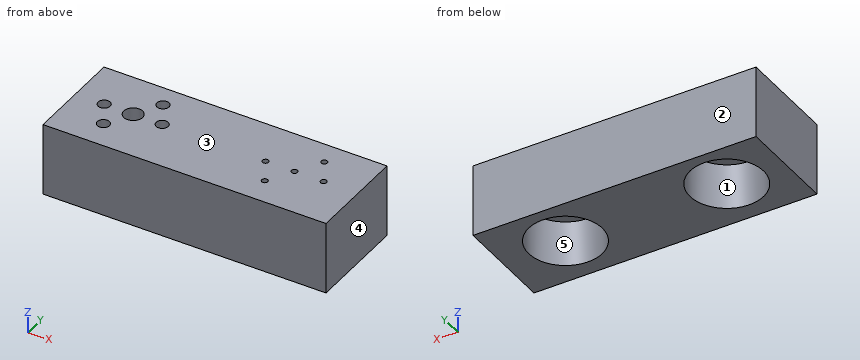
Autodesk Inventor part; units mm, degrees
ref_plane "YZ Plane" through (0, 0, 0) normal (1, 0, 0) x (0, 1, 0)
ref_plane "XZ Plane" through (0, 0, 0) normal (0, 1, 0) x (-1, 0, 0)
ref_plane "XY Plane" through (0, 0, 0) normal (0, 0, 1) x (1, 0, 0)
sketch "Sketch1" plane through (0, 0, 0) normal (0, 0, 1) x (1, 0, 0)
  circle A0 centre (49.887, 0) radius 0.7937
  circle A1 centre (34.647, 0) radius 0.7937
  circle A2 centre (42.267, 0) radius 9.525
  circle A3 centre (38.457, -6.5991) radius 0.7937
  circle A4 centre (46.077, 6.5991) radius 0.7937
  circle A5 centre (42.267, 0) radius 0.7937
  line L0 (-15.4509, 12.6033) -> (58.8878, 12.6033)
  line L1 (58.8878, 12.6033) -> (58.8878, -13.7292)
  line L2 (58.8878, -13.7292) -> (-15.4509, -13.7292)
  line L3 (-15.4509, -13.7292) -> (-15.4509, 12.6033)
  circle A6 centre (7.3609, 0.2473) radius 1.5875
  circle A7 centre (-7.8791, 0.2473) radius 1.5875
  circle A8 centre (-0.2591, 0.2473) radius 9.525
  circle A9 centre (3.5509, 6.8464) radius 1.5875
  circle A10 centre (-4.0691, -6.3518) radius 1.5875
  circle A11 centre (-0.2591, 0.2473) radius 2.4765
  circle A12 centre (42.267, 0) radius 9.652
  circle A13 centre (-0.2591, 0.2473) radius 9.652
  point P0 (37.5045, -8.2489)
  point P1 (47.0295, 8.2489)
  point P2 (-5.0216, -8.0016)
  point P3 (4.5034, 8.4962)
  dimension "d69" = 1.5875
  dimension "d70" = 1.5875
  dimension "d75" = 1.5875
  dimension "d76" = 1.5875
  dimension "d79" = 7.62
  dimension "d80" = 7.62
  dimension "d82" = 1.5875
  dimension "d83" = 7.62
  dimension "d84" = 7.62
  dimension "d85" = 3.175
  dimension "d86" = 3.175
  dimension "d87" = 3.175
  dimension "d88" = 3.175
  dimension "d89" = 7.62
  dimension "d90" = 7.62
  dimension "d91" = 4.953
  dimension "d92" = 7.62
  dimension "d93" = 7.62
  dimension "d95" = 19.304
  dimension "d96" = 19.304
extrude "Extrusion14" add sketch "Sketch1" along normal blind 19.05 contours A2 | L0 L1 L2 L3 | A8 | A12 | A13
extrude "Extrusion15" cut sketch "Sketch1" along normal blind 11.938 contours A0 | A1 | A2 | A3 | A4 | A5 | A6 | A7 | A8 | A9 | A10 | A11 | A12 | A13
properties part number "C.Crank Connect Shaft Cutting Jig"
For this review, take the finished solid that the model builds, in its own axes (mm). Face numbers are marked on the shaded views. A direction names the side the tool comes from. Coordinates: 2 decimals unless noted, no trailing zeros. Write each loop counter-clockwise with the first axis right and the second up, starting at its lowest first coordinate (ties: lowest second). Pieces come first, ordered by that corner, then holes. Notation, with made-up numbers: (28, 58) - (75, 58) arc R3 cw to (75, 63) - close; hole circle Ø7 at (17.25, 89). An arc over 180 degrees is marked (long way). Answer in a Markdown table with one row per item. Add a question column.
Q1. We need section D-D, the plane x = 44.5. State the section outline as (y, z) points.
Q2. Tool access review of the marked faces 1 and 2: name each direction out of +Z, -Z, +X, -X, +Y, -Y from which nothing blocks a thin tool from reaching the whole face with its end or side.
Q3. We need section A-A, the plane z = 15. Count the separate pieces of the cut face and the enclosed holes in it, and give its area (3 significant figures).
Q4. Draft analysis for pull direction X (two halves, no side actions). For the marked faces 3, 4 and 5, state which applies: +X half, -X half, draft (parallel to the pull), parting line (faces both ways), or undercut.
Q5. For P1, Ø4, axis at x = 7.36, y = 0.25, coming from the -Z side, flat-tipped, find the tip position at first contact; note if it passes through.
Q6. We need section B-B, the plane x = 0.5. State the section outline as (y, z) points.
Q7. We need section C-C, the plane z = 9. State the section outline as (x, y) points.
Q8. For probe 1 along X at (y, z) = (1.5, 12.5); probe 2 along Y at (x, z) = (3.5, 13.5); probe 3 along X at (y, z) = (5, 1), list the stretches that pass through material, from the lowest coordinate up.
Answer list:
| question | item | result |
|---|---|---|
| 1 | outline | (-13.73, 0) - (-9.39, 0) - (-9.39, 11.94) - (9.39, 11.94) - (9.39, 0) - (12.6, 0) - (12.6, 19.05) - (-13.73, 19.05) - close |
| 2 | face 1 | -Z |
| 2 | face 2 | +Z, -Z, +X, -X, +Y |
| 3 | separate pieces | 1 |
| 3 | enclosed holes | 10 |
| 3 | area | 1,900 mm2 |
| 4 | face 3 | draft |
| 4 | face 4 | +X half |
| 4 | face 5 | undercut |
| 5 | P1 | stops at z = 11.94 |
| 6 | outline | (-13.73, 0) - (-9.37, 0) - (-9.37, 11.94) - (-2.11, 11.94) - (-2.11, 19.05) - (-13.73, 19.05) - close; (2.6, 11.94) - (9.87, 11.94) - (9.87, 0) - (12.6, 0) - (12.6, 19.05) - (2.6, 19.05) - close |
| 7 | outline | (-15.45, -13.73) - (58.89, -13.73) - (58.89, 12.6) - (-15.45, 12.6) - close; hole circle Ø19.3 at (-0.26, 0.25); hole circle Ø19.3 at (42.27, 0) |
| 8 | probe 1 | x = -15.45 to -8.85, -6.9 to -2.4, 1.88 to 6.39, 8.34 to 58.89 |
| 8 | probe 2 | y = -13.73 to 5.26, 8.43 to 12.6 |
| 8 | probe 3 | x = -15.45 to -8.66, 8.14 to 34.01, 50.52 to 58.89 |
